For this review, take the finished solid that the model builds, in its own axes (mm). A direction names the side the tool comes from. Coordinates: 2 decimals unless noted, no trailing zeros. Order: outer loops, then holes, each group sorted by start corner. A loop starts at its lowest first (then second) coordinate and runs counter-clockwise, first axis right, second up. Notation, with made-up numbers: (-30, 21.5) -> (12, 21.5) arc R26 ccw to (12, 44.5) -> close; hole circle Ø6 at (9.25, 82.5). An arc over 180 degrees is marked (long way). Write item = value, one per line. Start each with the question number.
1) Draft analysis for pull direction Y (two halves, no side actions). For faces 4 (the face through (10.12, -1.98, 1.68)), 5 (the face through (8, 7, -10)), 6 (the face through (4, 0, 0)), state which applies: +Y half, -Y half, draft (parallel to the pull), parting line (faces both ways), or undercut.
2) Insertion check: pin 1 Ø5 at (x, y) = (8, 1.5) entering from -Z; pin 2 Ø5 at (x, z) = (6, -18) entering from -Y; pin 3 Ø5.5 at (x, y) = (7.54, 0) entering from -Z. Each pin has a flat end and moves straight along its axis. Give the tip position at first contact, or say it passes through.
3) Consider section D-D on z = -6. Give the boundary of the cut face in (x, y).
4) Consider section B-B on x = 4.75. Give the boundary of the cut face in (y, z), and give its area (3 significant figures).
5) Consider section A-A on y = 0. Give the boundary of the cut face in (x, z), and give its area (3 significant figures).
6) Machinability: for faces 1 (the face through (8, 5, -12)), 2 (the face through (8, 6, -25)), 3 (the face through (6.1, -1.4, 3.4)), which of the approach directions +Z, -Z, +X, -X, +Y, -Y give a long, thin tool a straight path to every point of the face, cutting with its end or side? Answer none if there is none.
7) Consider section C-C on y = 4. Give the boundary of the cut face in (x, z), and give its area (3 significant figures).
8) Wall thickness on probe 1 along Z at (x, y) = (4.5, 3.5); probe 2 along Z at (x, y) = (6.75, 2.25); probe 3 along Y at (x, z) = (2, -1.75): over which ranges is each line inside the solid? List them lowest first. Write a range as [from, to].
from build123d import *

# Parameters (mm, degrees)
SKETCH_1_W                   = 15
SKETCH_1_H                   = 12
EXTRUDE_1_DEPTH              = 5
SKETCH_2_W                   = 15
SKETCH_2_H                   = 2
EXTRUDE_2_DEPTH              = 25
SKETCH_6_W                   = 15
SKETCH_6_H                   = 5
CUT_EXTRUDE_2_DEPTH          = 6
SKETCH_7_W                   = 15
SKETCH_7_H                   = 5
EXTRUDE_3_DEPTH              = 5
HOLE_WIZARD_M3_1_D           = 3.4
HOLE_WIZARD_M3_1_DEPTH       = 7.5
HOLE_WIZARD_M3_1_CBORE_D     = 6.5
HOLE_WIZARD_M3_1_CBORE_DEPTH = 3.4
HOLE_WIZARD_M3_1_TIP         = 1.021463052


with BuildPart() as part:
    # 草图1 → 凸台-拉伸1 (new body)
    with BuildSketch(Plane.XY):
        with Locations((7.5, 6)):
            Rectangle(SKETCH_1_W, SKETCH_1_H)
    extrude(amount=EXTRUDE_1_DEPTH)

    # 草图2 → 凸台-拉伸2 (add)
    with BuildSketch(Plane(origin=(0, 0, 0), x_dir=(-1, 0, 0), z_dir=(0, 0, -1))):
        with Locations((-7.5, 6)):
            Rectangle(SKETCH_2_W, SKETCH_2_H)
    extrude(amount=EXTRUDE_2_DEPTH)

    # 草图6 → 切除-拉伸2 (cut, through all)
    with BuildSketch(Plane(origin=(0, 0, 0), x_dir=(-1, 0, 0), z_dir=(0, 0, -1))):
        with Locations((-7.5, 9.5)):
            Rectangle(SKETCH_6_W, SKETCH_6_H)
    extrude(amount=-CUT_EXTRUDE_2_DEPTH, mode=Mode.SUBTRACT)

    # 草图7 → 凸台-拉伸3 (add)
    with BuildSketch(Plane.XZ):
        with Locations((7.5, 2.5)):
            Rectangle(SKETCH_7_W, SKETCH_7_H)
    extrude(amount=EXTRUDE_3_DEPTH)

    # M3 六角凹头螺钉的柱形沉头孔1
    with Locations(Plane(origin=(0, 0, 0), x_dir=(-1, 0, 0), z_dir=(0, 0, -1))):
        with Locations((-7.544327116, 0)):
            CounterBoreHole(HOLE_WIZARD_M3_1_D / 2, HOLE_WIZARD_M3_1_CBORE_D / 2, HOLE_WIZARD_M3_1_CBORE_DEPTH, depth=HOLE_WIZARD_M3_1_DEPTH)
            with Locations((0, 0, -(HOLE_WIZARD_M3_1_DEPTH + HOLE_WIZARD_M3_1_TIP / 2))):  # 118° drill point
                Cone(0, HOLE_WIZARD_M3_1_D / 2, HOLE_WIZARD_M3_1_TIP, mode=Mode.SUBTRACT)


solid = part.part
Answer sheet:
q1.face_4 = undercut
q1.face_5 = +Y half
q1.face_6 = draft
q2.pin_1 = 0
q2.pin_2 = 5
q2.pin_3 = 3.4
q3.outline = (0, 5) -> (15, 5) -> (15, 7) -> (0, 7) -> close
q4.outline = (-5, 0) -> (-1.66, 0) -> (-1.66, 3.4) -> (1.66, 3.4) -> (1.66, 0) -> (5, 0) -> (5, -25) -> (7, -25) -> (7, 5) -> (-5, 5) -> close
q4.area = 98.7 mm2
q5.outline = (0, 0) -> (4.29, 0) -> (4.29, 3.4) -> (5.84, 3.4) -> (5.84, 5) -> (0, 5) -> close; (9.24, 3.4) -> (10.79, 3.4) -> (10.79, 0) -> (15, 0) -> (15, 5) -> (9.24, 5) -> close
q5.area = 47.5 mm2
q6.face_1 = -Z, +X, -X, -Y
q6.face_2 = -Z, +X, -X, +Y, -Y
q6.face_3 = -Z
q7.outline = (0, 0) -> (15, 0) -> (15, 5) -> (0, 5) -> close
q7.area = 75.0 mm2
q8.probe_1 = [0, 5]
q8.probe_2 = [3.4, 5]
q8.probe_3 = [5, 7]
